from build123d import *

# Parameters (mm, degrees)
F_1_FR_W               = 149.275698602
F_1_FR_H               = 51.18023952
SM_BASE_FLANGE_1_DEPTH = 3


# Sheet-metal steps are written as plain solids
with BuildPart() as part:
    # Эскиз1_fr → Базовая кромка1 (new body)
    with BuildSketch(Plane.XY):
        Rectangle(F_1_FR_W, F_1_FR_H)
        Polygon((39.926451229, -10.672105555), (-39.926451229, -10.672105555), (-39.926451229, 10.672105555), (39.926451229, 10.672105555), (39.926451229, 6.791965083), (-25.410080628, 6.791965083), (-25.410080628, -3.177311756), (-21.795427302, -6.791965083), (39.926451229, -6.791965083), align=None, mode=Mode.SUBTRACT)
    extrude(amount=-SM_BASE_FLANGE_1_DEPTH)


solid = part.part
Source: CAD feature listing. Evaluate the final solid. Frame: model axes, mm. A direction names the side the tool comes from. Give positions to 0.01 mm unless a question says otherwise; leave off trailing zeros. Write each loop counter-clockwise with the first axis right and the second up, starting at its lowest first coordinate (ties: lowest second). Pieces come first, ordered by that corner, then holes. Notation, with made-up numbers: M 9,2 L 59,2 A12 ccw 59,12 Z; hole C 39.5,44 d7. An arc over 180 degrees is marked long. Return JSON: item names as keys, results as strings. Group by question number.
1) Cut plane A-A, the plane x = 22. Output: boundary loops of the cut face in (y, z), then the cut area to 3 significant figures.
2) Cut plane C-C, the plane z = -0.6. Output: boundary loops of the cut face in (x, y), then the cut area to 3 significant figures.
3) Cut plane B-B, the plane y = 5.5. Output: boundary loops of the cut face in (x, z).
4) Set-up query: faces 5 (the face through (-1, 25.59, -1)), 6 (the face through (1, -10.672, -1)). Return all of +Z, -Z, +X, -X, +Y, -Y with unobstructed straight access to the full face (end or side cutting, diameter ignored); none if empty.
5) Ray query, L1, parallel to Y at x = 34, z = -2.5; L2, parallel to X at y = -7, z = -2.9; L3, parallel to Y at x = -38.5, z = -2.35. Return the intervals inside material, ascending.
6) Cut plane D-D, the plane x = -34. Output: boundary loops of the cut face in (y, z), then the cut area to 3 significant figures.
7) Draft query along X for faces 1 (the face through (-74.638, 0, -1)), 2 (the face through (8, 6.792, -1)), 3 (the face through (74.638, 0, -1)), 4 (the face through (-1, -25.59, -1)). Return one class per face: released by +X, released by -X, zero draft, split by the parting line, or undercut.
Data:
{
 "1": {"outline": "M -25.59,-3 L -10.67,-3 L -10.67,0 L -25.59,0 Z; M -6.79,-3 L 6.79,-3 L 6.79,0 L -6.79,0 Z; M 10.67,-3 L 25.59,-3 L 25.59,0 L 10.67,0 Z", "area": "130 mm²"},
 "2": {"outline": "M -74.64,-25.59 L 74.64,-25.59 L 74.64,25.59 L -74.64,25.59 Z; hole M -39.93,-10.67 L 39.93,-10.67 L 39.93,-6.79 L -21.8,-6.79 L -25.41,-3.18 L -25.41,6.79 L 39.93,6.79 L 39.93,10.67 L -39.93,10.67 Z", "area": "6,820 mm²"},
 "3": {"outline": "M -74.64,-3 L -39.93,-3 L -39.93,0 L -74.64,0 Z; M -25.41,-3 L 74.64,-3 L 74.64,0 L -25.41,0 Z"},
 "4": {"face 5": "+Z, -Z, +X, -X, +Y", "face 6": "+Z, -Z"},
 "5": {"L1": "y = -25.59 to -10.67, -6.79 to 6.79, 10.67 to 25.59", "L2": "x = -74.64 to -39.93, 39.93 to 74.64", "L3": "y = -25.59 to -10.67, 10.67 to 25.59"},
 "6": {"outline": "M -25.59,-3 L -10.67,-3 L -10.67,0 L -25.59,0 Z; M 10.67,-3 L 25.59,-3 L 25.59,0 L 10.67,0 Z", "area": "89.5 mm²"},
 "7": {"face 1": "released by -X", "face 2": "undercut", "face 3": "released by +X", "face 4": "zero draft"}
}
